```python
from build123d import *

# Parameters (mm, degrees)
F2_R     = 25.4
F3_DEPTH = 12.7
F4_R     = 3.175
F5_DEPTH = 25.4
F6_R     = 3.9751
F7_DEPTH = 10.16
F8_R     = 1.7272
F9_DEPTH = 70.55837


with BuildPart() as f1:
    # F0 (on Front) → F1 (revolve)
    with BuildSketch(Plane.XZ):
        Polygon((-51.577873, 29.3751), (-51.577873, 0), (-26.177873, 0), (-26.177873, 30.1625), (-40.909873, 30.1625), (-40.909873, 29.3751), align=None)
    revolve(axis=Axis((-38.877873, 0, 0), (-1, 0, 0)))

    # F2 (on face) → F3 (cut)
    with BuildSketch(Plane.YZ.offset(-26.177873)):
        Circle(F2_R)
    extrude(amount=-F3_DEPTH, mode=Mode.SUBTRACT)

    # F4 (on face) → F5 (cut)
    with BuildSketch(Plane(origin=(-51.577873, 0, 0), x_dir=(0, -1, 0), z_dir=(-1, 0, 0))):
        Circle(F4_R)
    extrude(amount=-F5_DEPTH, mode=Mode.SUBTRACT)

    # F6 (on face) → F7 (cut)
    with BuildSketch(Plane(origin=(-51.577873, 0, 0), x_dir=(0, -1, 0), z_dir=(-1, 0, 0))):
        with Locations((0, 21.1455)):
            Circle(F6_R)
    extrude(amount=-F7_DEPTH, mode=Mode.SUBTRACT)

    # F8 (on Front) → F9 (cut)
    with BuildSketch(Plane.XZ):
        with Locations((-48.098073, 0)):
            Circle(F8_R)
    extrude(amount=-F9_DEPTH, mode=Mode.SUBTRACT)


solid = f1.part
```
Here's how the part is built. I have some questions about the finished solid (model axes, mm). A direction names the side the tool comes from. Coordinates: 2 decimals unless noted, no trailing zeros. Order: outer loops, then holes, each group sorted by start corner. A loop starts at its lowest first (then second) coordinate and runs counter-clockwise, first axis right, second up.
Item 1: Thinking about a two-plate mould opening in X: for faces 1 (the face through (-46.45, 15.83, 0.52)), 2 (the face through (-26.178, -20, 16)), 3 (the face through (-40.91, -29, 7)), which applies, pulls with the +X half, pulls with the -X half, needs draft (parallel to the pull), parting line crosses it, or undercut?
Response values:
face 1: undercut
face 2: pulls with the +X half
face 3: pulls with the -X half
Item 2: If we section it at B-B, the plane z = 0: List the corners of the cut face in (x, y) for me (1 decimal), then the cut area to 3 significant figures.
Response values:
outline: (-51.6, -29.4) - (-40.9, -29.4) - (-40.9, -30.2) - (-26.2, -30.2) - (-26.2, -25.4) - (-38.9, -25.4) - (-38.9, -3.2) - (-51.6, -3.2) - close; (-51.6, 3.2) - (-49.8, 3.2) - (-49.8, 29.4) - (-51.6, 29.4) - close; (-46.4, 3.2) - (-38.9, 3.2) - (-38.9, 25.4) - (-26.2, 25.4) - (-26.2, 30.2) - (-40.9, 30.2) - (-40.9, 29.4) - (-46.4, 29.4) - close
area: 699 mm2
Item 3: If we section it at D-D, the plane z = -11.5: List the corners of the cut face in (x, y) for me.
Response values:
outline: (-51.58, -27.03) - (-40.91, -27.03) - (-40.91, -27.88) - (-26.18, -27.88) - (-26.18, -22.65) - (-38.88, -22.65) - (-38.88, 22.65) - (-26.18, 22.65) - (-26.18, 27.88) - (-40.91, 27.88) - (-40.91, 27.03) - (-51.58, 27.03) - close
Item 4: If we section it at C-C, the plane y = 11: List the corners of the cut face in (x, z) for me, then the cut area to 3 significant figures.
Response values:
outline: (-51.58, -27.24) - (-40.91, -27.24) - (-40.91, -28.09) - (-26.18, -28.09) - (-26.18, -22.89) - (-38.88, -22.89) - (-38.88, 22.89) - (-26.18, 22.89) - (-26.18, 28.09) - (-40.91, 28.09) - (-40.91, 27.24) - (-51.58, 27.24) - close; hole circle Ø3.45 at (-48.1, 0)
area: 818 mm2
Item 5: Which directions (+Z, -Z, +X, -X, +Y, -Y) give clear straight access to the entire face, cutting with the end or side of a thin tool? Please do faces 4 (the face through (-33.647, 1.326, -30.133)), 5 (the face through (-32.439, -5.506, -24.796)), 6 (the face through (-46.569, 0.517, 25.087)).
Response values:
face 4: +X, -X
face 5: +X
face 6: -X
Item 6: I need wall thicknesses on probe 1 along Y at (x, z) = (-42.25, 0) (3 decimals); probe 2 along X at (y, z) = (4.5, -13); probe 3 along X at (y, z) = (19.25, 0). Which ranges of each line are inside material? Lowest first, please.
Response values:
probe 1: y = -29.375 to -3.175, 3.175 to 29.375
probe 2: x = -51.58 to -38.88
probe 3: x = -51.58 to -49.83, -46.37 to -38.88
Item 7: If we section it at A-A, the plane y = 0: List the corners of the cut face in (x, z) for me (1 decimal).
Response values:
outline: (-51.6, -29.4) - (-40.9, -29.4) - (-40.9, -30.2) - (-26.2, -30.2) - (-26.2, -25.4) - (-38.9, -25.4) - (-38.9, -3.2) - (-51.6, -3.2) - close; (-51.6, 3.2) - (-38.9, 3.2) - (-38.9, 25.4) - (-26.2, 25.4) - (-26.2, 30.2) - (-40.9, 30.2) - (-40.9, 29.4) - (-51.6, 29.4) - (-51.6, 25.1) - (-41.4, 25.1) - (-41.4, 17.2) - (-51.6, 17.2) - close
Item 8: I'm going to push flat-ended pins straight in: pin 1 Ø15 at (y, z) = (-8.5, -1.5) entering from +X; pin 2 Ø4 at (x, y) = (-33, -7.5) entering from +Z; pin 3 Ø5 at (x, y) = (-44.5, -4.5) entering from -Z. Where does each tip first touch, or does it pass through?
Response values:
pin 1: stops at x = -38.88
pin 2: stops at z = 29.66
pin 3: stops at z = -29.31
